from build123d import *

# Parameters (mm, degrees)
SKETCH1_W           = 129
SKETCH1_H           = 74
BOSS_EXTRUDE1_DEPTH = 4
SKETCH4_W           = 4
SKETCH4_H           = 10
SKETCH4_W_2         = 10
SKETCH4_H_2         = 4
CUT_EXTRUDE3_DEPTH  = 5
SKETCH5_W           = 135
SKETCH5_H           = 80
SKETCH5_W_2         = 129
SKETCH5_H_2         = 74
BOSS_EXTRUDE2_DEPTH = 4
SKETCH6_W           = 10
SKETCH6_H           = 20
SKETCH6_R           = 1.75
BOSS_EXTRUDE3_DEPTH = 4
FILLET1_R           = 4


with BuildPart() as part:
    # Sketch1 → Boss-Extrude1 (new body)
    with BuildSketch(Plane(origin=(0, 0, 0), x_dir=(1, 0, 0), z_dir=(0, 1, 0))):
        with Locations((64.5, -37)):
            Rectangle(SKETCH1_W, SKETCH1_H)
    extrude(amount=BOSS_EXTRUDE1_DEPTH)

    # Sketch4 → Cut-Extrude3 (cut, through all)
    with BuildSketch(Plane(origin=(0, 4, 0), x_dir=(1, 0, 0), z_dir=(0, 1, 0))):
        with Locations((127, -57)):
            Rectangle(SKETCH4_W, SKETCH4_H)
        with Locations((127, -37)):
            Rectangle(SKETCH4_W, SKETCH4_H)
        with Locations((127, -17)):
            Rectangle(SKETCH4_W, SKETCH4_H)
        with Locations((2, -57)):
            Rectangle(SKETCH4_W, SKETCH4_H)
        with Locations((2, -37)):
            Rectangle(SKETCH4_W, SKETCH4_H)
        with Locations((2, -17)):
            Rectangle(SKETCH4_W, SKETCH4_H)
        with Locations((104.5, -2)):
            Rectangle(SKETCH4_W_2, SKETCH4_H_2)
        with Locations((84.5, -2)):
            Rectangle(SKETCH4_W_2, SKETCH4_H_2)
        with Locations((64.5, -2)):
            Rectangle(SKETCH4_W_2, SKETCH4_H_2)
        with Locations((44.5, -2)):
            Rectangle(SKETCH4_W_2, SKETCH4_H_2)
        with Locations((24.5, -2)):
            Rectangle(SKETCH4_W_2, SKETCH4_H_2)
        with Locations((104.5, -72)):
            Rectangle(SKETCH4_W_2, SKETCH4_H_2)
        with Locations((84.5, -72)):
            Rectangle(SKETCH4_W_2, SKETCH4_H_2)
        with Locations((64.5, -72)):
            Rectangle(SKETCH4_W_2, SKETCH4_H_2)
        with Locations((44.5, -72)):
            Rectangle(SKETCH4_W_2, SKETCH4_H_2)
        with Locations((24.5, -72)):
            Rectangle(SKETCH4_W_2, SKETCH4_H_2)
    extrude(amount=-CUT_EXTRUDE3_DEPTH, mode=Mode.SUBTRACT)

    # Sketch5 → Boss-Extrude2 (add, through all)
    with BuildSketch(Plane(origin=(0, 4, 0), x_dir=(1, 0, 0), z_dir=(0, 1, 0))):
        with Locations((64.5, -37)):
            Rectangle(SKETCH5_W, SKETCH5_H)
        with Locations((64.5, -37)):
            Rectangle(SKETCH5_W_2, SKETCH5_H_2, mode=Mode.SUBTRACT)
    extrude(amount=-BOSS_EXTRUDE2_DEPTH)

    # Sketch6 → Boss-Extrude3 (add, through all)
    with BuildSketch(Plane.XZ):
        with Locations((137, 37)):
            Rectangle(SKETCH6_W, SKETCH6_H)
        with Locations((137, 37)):
            Circle(SKETCH6_R, mode=Mode.SUBTRACT)
        with Locations((-8, 37)):
            Rectangle(SKETCH6_W, SKETCH6_H)
        with Locations((-8, 37)):
            Circle(SKETCH6_R, mode=Mode.SUBTRACT)
    extrude(amount=-BOSS_EXTRUDE3_DEPTH)

    # Fillet1
    fillet1_edges = [part.edges().sort_by_distance(p)[0] for p in [
        (132, 2, -3),
        (132, 2, 77),
        (-3, 2, 77),
        (-3, 2, -3),
        (132, 2, 27),
        (132, 2, 47),
        (142, 2, 47),
        (142, 2, 27),
        (-13, 2, 27),
        (-13, 2, 47),
        (-3, 2, 47),
        (-3, 2, 27),
    ]]
    fillet(fillet1_edges, radius=FILLET1_R)


solid = part.part
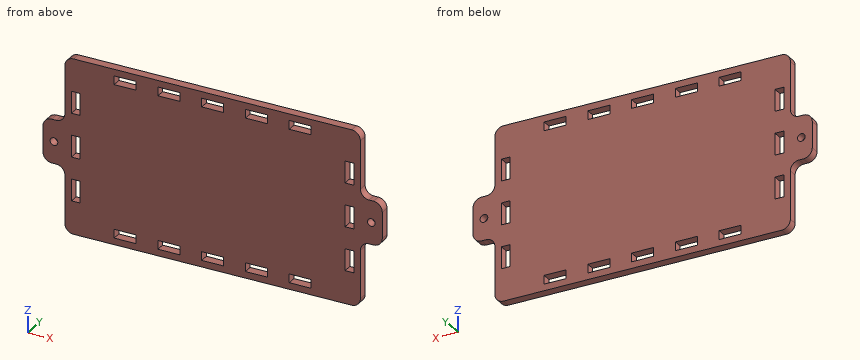
Input: part model. Units: mm. Frame: model coordinates. Round coordinates to 2 decimals unless told otherwise and drop trailing zeros. Order: outer loops, then holes, each group sorted by start corner. A loop starts at its lowest first (then second) coordinate and runs counter-clockwise, first axis right, second up. Notation, with made-up numbers: (88, 69.25) - (113, 69.25) arc R35 cw to (113, 105.25) - close; hole circle Ø10 at (-3.5, -31). An arc over 180 degrees is marked (long way). Answer as a JSON object with one key per item and string values. Group by question number.
(1) Cut plane D-D (y = 2.8). Count the separate pieces of the cut face and the enclosed holes in it, then the cut area to 3 significant figures.
(2) Pin query (flat end, axial travel): P1, Ø2, axis at y = 2, z = 55, coming from the -X side; P2, Ø1.5, axis at y = 0.5, z = 47, coming from the -X side; P3, Ø2, axis at x = -7.5, y = 3, coming from the -Z side. Return the tip coordinate at first contact, or that it passes through.
(3) Cut plane A-A (z = 37). Return loops of the section in (x, y), then the cut area to 3 significant figures.
(4) Cut plane B-B (x = 61.5). Return loops of the section in (y, z), then the cut area to 3 significant figures.
(5) Cut plane C-C (z = 17). Return loops of the section in (x, y), then the cut area to 3 significant figures.
(6) Material intervals for probe 1 along X at (y, z) = (3, 53.5); probe 2 along Z at (x, y) = (48.5, 1.35); probe 3 along X at (y, z) = (1.25, 72.5), sorted ascending. Write a range as from..to.
Here are the results:
{
 "1": {"separate pieces": "1", "enclosed holes": "18", "area": "10,500 mm^2"},
 "2": {"P1": "stops at x = -3", "P2": "stops at x = -11.33", "P3": "stops at z = 26.97"},
 "3": {"outline": "(-13, 0) - (-9.75, 0) - (-9.75, 4) - (-13, 4) - close; (-6.25, 0) - (0, 0) - (0, 4) - (-6.25, 4) - close; (4, 0) - (125, 0) - (125, 4) - (4, 4) - close; (129, 0) - (135.25, 0) - (135.25, 4) - (129, 4) - close; (138.75, 0) - (142, 0) - (142, 4) - (138.75, 4) - close", "area": "560 mm^2"},
 "4": {"outline": "(0, -3) - (4, -3) - (4, 0) - (0, 0) - close; (0, 4) - (4, 4) - (4, 70) - (0, 70) - close; (0, 74) - (4, 74) - (4, 77) - (0, 77) - close", "area": "288 mm^2"},
 "5": {"outline": "(-3, 0) - (0, 0) - (0, 4) - (-3, 4) - close; (4, 0) - (125, 0) - (125, 4) - (4, 4) - close; (129, 0) - (132, 0) - (132, 4) - (129, 4) - close", "area": "508 mm^2"},
 "6": {"probe 1": "x = -3..0, 4..125, 129..132", "probe 2": "z = -3..0, 4..70, 74..77", "probe 3": "x = -3..19.5, 29.5..39.5, 49.5..59.5, 69.5..79.5, 89.5..99.5, 109.5..132"}
}
